from build123d import *

# Parameters (mm, degrees)
SKETCH_1_W           = 20
SKETCH_1_H           = 30
SKETCH_1_W_2         = 18
SKETCH_1_H_2         = 28
EXTRUDE_1_DEPTH      = 600
SKETCH_2_R           = 1.55
SKETCH_2_R_2         = 3
CUT_EXTRUDE_1_DEPTH  = 5
SKETCH_5_R           = 5
CUT_EXTRUDE_6_DEPTH  = 10
SKETCH_7_R           = 1.25
CUT_EXTRUDE_7_DEPTH  = 25
SKETCH_8_R           = 4
CUT_EXTRUDE_8_DEPTH  = 3
SKETCH_10_R          = 1.6
CUT_EXTRUDE_9_DEPTH  = 40
SKETCH_11_R          = 2.5
CUT_EXTRUDE_10_DEPTH = 40
SKETCH_13_R          = 2.5
CUT_EXTRUDE_11_DEPTH = 40
CUT_EXTRUDE_12_DEPTH = 10
SKETCH_16_R          = 2.5
CUT_EXTRUDE_13_DEPTH = 50
SKETCH_17_R          = 2.5
CUT_EXTRUDE_14_DEPTH = 50
SKETCH_18_R          = 1.55
CUT_EXTRUDE_15_DEPTH = 40
SKETCH_19_R          = 1.55
CUT_EXTRUDE_16_DEPTH = 40
SKETCH_20_R          = 10
CUT_EXTRUDE_17_DEPTH = 40


with BuildPart() as part:
    # 草图1 → 凸台-拉伸1 (new body)
    with BuildSketch(Plane.XY):
        Rectangle(SKETCH_1_W, SKETCH_1_H)
        Rectangle(SKETCH_1_W_2, SKETCH_1_H_2, mode=Mode.SUBTRACT)
    extrude(amount=EXTRUDE_1_DEPTH)

    # 草图2 → 切除-拉伸1 (cut)
    with BuildSketch(Plane(origin=(0, 15, 0), x_dir=(1, 0, 0), z_dir=(0, 1, 0))):
        with Locations(Location((0, -217.88, 0), (0, 0, 270))):
            Circle(SKETCH_2_R)
        with Locations(Location((0, -235.88, 0), (0, 0, 270))):
            Circle(SKETCH_2_R)
        with Locations(Location((0, -367.88, 0), (0, 0, 270))):
            Circle(SKETCH_2_R)
        with Locations(Location((0, -385.88, 0), (0, 0, 270))):
            Circle(SKETCH_2_R)
        with Locations(Location((0, -301.88, 0), (0, 0, 270))):
            Circle(SKETCH_2_R_2)
    extrude(amount=-CUT_EXTRUDE_1_DEPTH, mode=Mode.SUBTRACT)

    # 草图5 → 切除-拉伸6 (cut)
    with BuildSketch(Plane(origin=(0, -14, 0), x_dir=(1, 0, 0), z_dir=(0, 1, 0))):
        with Locations(Location((0, -385.88, 0), (0, 0, 270))):
            Circle(SKETCH_5_R)
        with Locations(Location((0, -367.88, 0), (0, 0, 270))):
            Circle(SKETCH_5_R)
        with Locations(Location((0, -235.88, 0), (0, 0, 270))):
            Circle(SKETCH_5_R)
        with Locations(Location((0, -217.88, 0), (0, 0, 270))):
            Circle(SKETCH_5_R)
    extrude(amount=-CUT_EXTRUDE_6_DEPTH, mode=Mode.SUBTRACT)

    # 草图7 → 切除-拉伸7 (cut)
    with BuildSketch(Plane(origin=(10, 0, 0), x_dir=(0, 0, -1), z_dir=(1, 0, 0))):
        with BuildLine():
            ThreePointArc((-587, -6.1), (-587.585786438, -4.685786438), (-589, -4.1))
            Line((-589, -4.1), (-589, -8.1))
            ThreePointArc((-589, -8.1), (-587.585786438, -7.514213562), (-587, -6.1))
        make_face()
        with BuildLine():
            Line((-589, -8.1), (-589, -4.1))
            ThreePointArc((-589, -4.1), (-591, -6.1), (-589, -8.1))
        make_face()
        with BuildLine():
            Line((-562, -4.1), (-589, -4.1))
            ThreePointArc((-589, -4.1), (-587.585786438, -4.685786438), (-587, -6.1))
            ThreePointArc((-587, -6.1), (-587.585786438, -7.514213562), (-589, -8.1))
            Line((-589, -8.1), (-562, -8.1))
            ThreePointArc((-562, -8.1), (-564, -6.1), (-562, -4.1))
        make_face()
        with Locations((-595, 6)):
            Circle(SKETCH_7_R)
        with BuildLine():
            ThreePointArc((-560, -6.1), (-560.585786438, -4.685786438), (-562, -4.1))
            Line((-562, -4.1), (-562, -8.1))
            ThreePointArc((-562, -8.1), (-560.585786438, -7.514213562), (-560, -6.1))
        make_face()
        with BuildLine():
            Line((-562, -8.1), (-562, -4.1))
            ThreePointArc((-562, -4.1), (-564, -6.1), (-562, -8.1))
        make_face()
        with BuildLine():
            ThreePointArc((-39.76, -6.1), (-40.345786438, -4.685786438), (-41.76, -4.1))
            Line((-41.76, -4.1), (-41.76, -8.1))
            ThreePointArc((-41.76, -8.1), (-40.345786438, -7.514213562), (-39.76, -6.1))
        make_face()
        with BuildLine():
            Line((-41.76, -8.1), (-41.76, -4.1))
            ThreePointArc((-41.76, -4.1), (-43.76, -6.1), (-41.76, -8.1))
        make_face()
        with BuildLine():
            ThreePointArc((-14.76, -8.1), (-16.76, -6.1), (-14.76, -4.1))
            Line((-14.76, -4.1), (-41.76, -4.1))
            ThreePointArc((-41.76, -4.1), (-40.345786438, -4.685786438), (-39.76, -6.1))
            ThreePointArc((-39.76, -6.1), (-40.345786438, -7.514213562), (-41.76, -8.1))
            Line((-41.76, -8.1), (-14.76, -8.1))
        make_face()
        with BuildLine():
            ThreePointArc((-12.76, -6.1), (-13.345786438, -4.685786438), (-14.76, -4.1))
            Line((-14.76, -4.1), (-14.76, -8.1))
            ThreePointArc((-14.76, -8.1), (-13.345786438, -7.514213562), (-12.76, -6.1))
        make_face()
        with BuildLine():
            Line((-14.76, -8.1), (-14.76, -4.1))
            ThreePointArc((-14.76, -4.1), (-16.76, -6.1), (-14.76, -8.1))
        make_face()
        with Locations((-575, 6)):
            Circle(SKETCH_7_R)
        with Locations((-8.76, 6)):
            Circle(SKETCH_7_R)
        with Locations((-28.76, 6)):
            Circle(SKETCH_7_R)
    extrude(amount=-CUT_EXTRUDE_7_DEPTH, mode=Mode.SUBTRACT)

    # 草图8 → 切除-拉伸8 (cut)
    with BuildSketch(Plane.ZY.offset(10)):
        with Locations((8.76, 6)):
            Circle(SKETCH_8_R)
        with Locations((28.76, 6)):
            Circle(SKETCH_8_R)
        with Locations((575, 6)):
            Circle(SKETCH_8_R)
        with Locations((595, 6)):
            Circle(SKETCH_8_R)
    extrude(amount=-CUT_EXTRUDE_8_DEPTH, mode=Mode.SUBTRACT)

    # 草图10 → 切除-拉伸9 (cut)
    with BuildSketch(Plane(origin=(0, 15, 0), x_dir=(1, 0, 0), z_dir=(0, 1, 0))):
        with Locations(Location((6, -585, 0), (0, 0, 270))):
            Circle(SKETCH_10_R)
        with Locations(Location((6, -565, 0), (0, 0, 270))):
            Circle(SKETCH_10_R)
        with Locations(Location((6, -38.76, 0), (0, 0, 270))):
            Circle(SKETCH_10_R)
        with Locations(Location((6, -18.76, 0), (0, 0, 270))):
            Circle(SKETCH_10_R)
    extrude(amount=-CUT_EXTRUDE_9_DEPTH, mode=Mode.SUBTRACT)

    # 草图11 → 切除-拉伸10 (cut)
    with BuildSketch(Plane.XZ.offset(15)):
        with Locations(Location((-3, 152, 0), (0, 0, 270))):
            Circle(SKETCH_11_R)
        with Locations(Location((-3, 172, 0), (0, 0, 270))):
            Circle(SKETCH_11_R)
    extrude(amount=-CUT_EXTRUDE_10_DEPTH, mode=Mode.SUBTRACT)

    # 草图13 → 切除-拉伸11 (cut)
    with BuildSketch(Plane.XZ.offset(15)):
        with Locations(Location((-3, 431.76, 0), (0, 0, 270))):
            Circle(SKETCH_13_R)
        with Locations(Location((-3, 451.76, 0), (0, 0, 270))):
            Circle(SKETCH_13_R)
    extrude(amount=-CUT_EXTRUDE_11_DEPTH, mode=Mode.SUBTRACT)

    # 草图14 → 切除-拉伸12 (cut)
    with BuildSketch(Plane(origin=(0, -14, 0), x_dir=(1, 0, 0), z_dir=(0, 1, 0))):
        with BuildLine():
            Line((6, -291.88), (6, -311.88))
            ThreePointArc((6, -311.88), (0, -317.88), (-6, -311.88))
            Line((-6, -311.88), (-6, -291.88))
            ThreePointArc((-6, -291.88), (0, -285.88), (6, -291.88))
        make_face()
    extrude(amount=-CUT_EXTRUDE_12_DEPTH, mode=Mode.SUBTRACT)

    # 草图16 → 切除-拉伸13 (cut)
    with BuildSketch(Plane.ZY.offset(10)):
        with Locations((464.88, 7)):
            Circle(SKETCH_16_R)
        with Locations((484.88, 7)):
            Circle(SKETCH_16_R)
    extrude(amount=-CUT_EXTRUDE_13_DEPTH, mode=Mode.SUBTRACT)

    # 草图17 → 切除-拉伸14 (cut)
    with BuildSketch(Plane.ZY.offset(10)):
        with Locations((118.88, 7)):
            Circle(SKETCH_17_R)
        with Locations((138.88, 7)):
            Circle(SKETCH_17_R)
    extrude(amount=-CUT_EXTRUDE_14_DEPTH, mode=Mode.SUBTRACT)

    # 草图18 → 切除-拉伸15 (cut)
    with BuildSketch(Plane(origin=(10, 0, 0), x_dir=(0, 0, -1), z_dir=(1, 0, 0))):
        with Locations((-28.76, -11)):
            Circle(SKETCH_18_R)
        with Locations((-8.76, -11)):
            Circle(SKETCH_18_R)
    extrude(amount=-CUT_EXTRUDE_15_DEPTH, mode=Mode.SUBTRACT)

    # 草图19 → 切除-拉伸16 (cut)
    with BuildSketch(Plane(origin=(10, 0, 0), x_dir=(0, 0, -1), z_dir=(1, 0, 0))):
        with Locations((-575, -11)):
            Circle(SKETCH_19_R)
        with Locations((-595, -11)):
            Circle(SKETCH_19_R)
    extrude(amount=-CUT_EXTRUDE_16_DEPTH, mode=Mode.SUBTRACT)

    # 草图20 → 切除-拉伸17 (cut)
    with BuildSketch(Plane.ZY.offset(10)):
        with Locations((81.88, 0)):
            Circle(SKETCH_20_R)
        with Locations((264.38, 0)):
            Circle(SKETCH_20_R)
        with Locations((339.38, 0)):
            Circle(SKETCH_20_R)
        with Locations((521.88, 0)):
            Circle(SKETCH_20_R)
    extrude(amount=-CUT_EXTRUDE_17_DEPTH, mode=Mode.SUBTRACT)


solid = part.part
Geometry: final body of the model. Coordinates: model frame, mm. A direction names the side the tool comes from. Give positions to 0.01 mm unless a question says otherwise; leave off trailing zeros. Order: outer loops, then holes, each group sorted by start corner. A loop starts at its lowest first (then second) coordinate and runs counter-clockwise, first axis right, second up. Notation, with made-up numbers: (-39.75, -17.5) -> (0.25, -17.5) arc R22 cw to (0.25, 17.5) -> close; hole circle Ø9 at (3.5, 73.5). An arc over 180 degrees is marked (long way). Put each result on its own line as item: value.
Q1. Reachability of faces 4 (the face through (9, 0, 296)), 5 (the face through (-9.51, 0.44, 71.89)), 6 (the face through (0.22, -14.493, 212.885)) from +Z, -Z, +X, -X, +Y, -Y: full face, straight path, thin tool, end or side. Return the list, or none.
Here are the results:
face 4: +Z, -Z
face 5: +X, -X
face 6: -Y
Q2. Material intervals for L1, parallel to X at y = -6, z = 193; L2, parallel to Y at x = -7.5, z = 507; L3, parallel to X at y = -14.8, z = 18.76, sorted ascending.
Here are the results:
L1: x = -10 to -9, 9 to 10
L2: y = -15 to -14, 14 to 15
L3: x = -10 to 4.4, 7.6 to 10
Q3. Section B-B, the plane z = 343. Return loops of the section in (x, y), then the cut area to 3 significant figures.
Here are the results:
outline: (-10, -15) -> (10, -15) -> (10, -9.32) -> (9, -9.32) -> (9, -14) -> (-9, -14) -> (-9, -9.32) -> (-10, -9.32) -> close; (-10, 9.32) -> (-9, 9.32) -> (-9, 14) -> (9, 14) -> (9, 9.32) -> (10, 9.32) -> (10, 15) -> (-10, 15) -> close
area: 58.7 mm^2
Q4. Draft query along Z for faces 1 (the face through (0, 15, 296)), 2 (the face through (-9.7, 0.1, 0)), 3 (the face through (-1.915, -14.493, 390.499)). Return one class per face: released by +Z, released by -Z, zero draft, split by the parting line, or undercut.
Here are the results:
face 1: zero draft
face 2: released by -Z
face 3: undercut
Q5. Section A-A, the plane z = 204. Return loops of the section in (x, y).
Here are the results:
outline: (-10, -15) -> (10, -15) -> (10, 15) -> (-10, 15) -> close; hole (-9, -14) -> (9, -14) -> (9, 14) -> (-9, 14) -> close
Q6. Pin query (flat end, axial travel): pin 1 (2 mm diameter, centred on x = 1, z = 234, fed in from -Y). Return the tip coordinate at first contact, or that it passes through.
Here are the results:
pin 1: stops at y = 14
